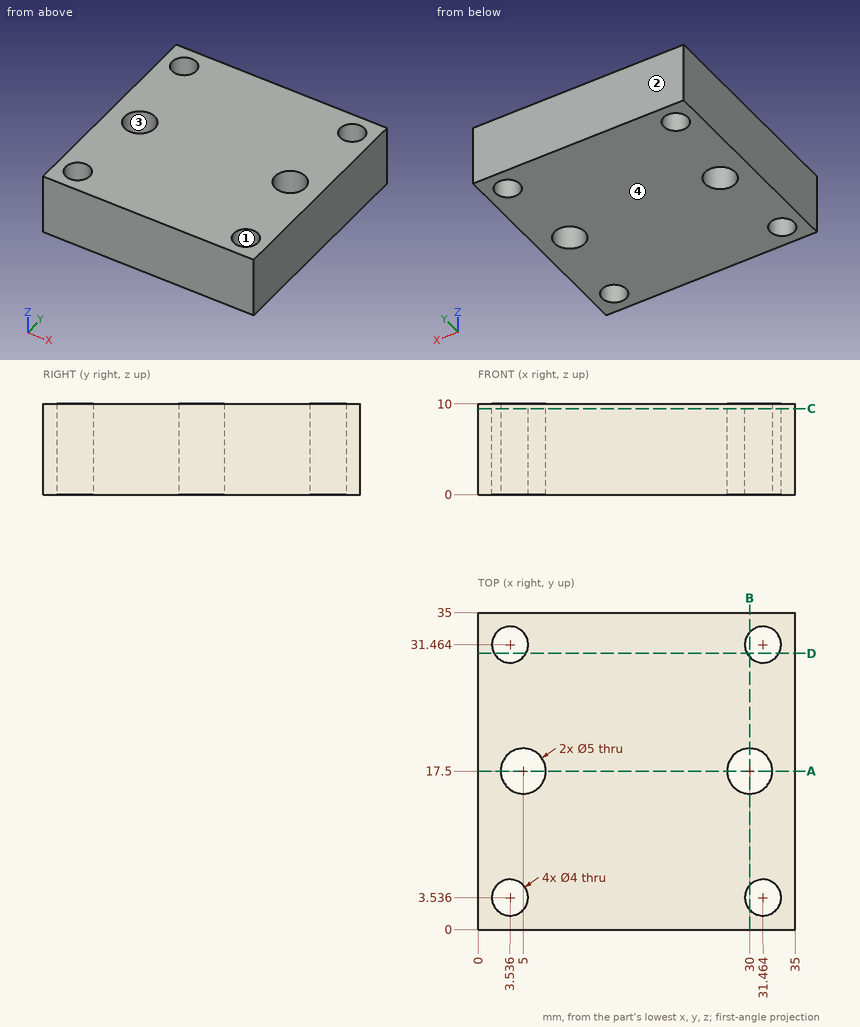
The figure shows three views and two pictorial views of one solid part (mm, origin at its lowest corner). Answer the questions. Give positions to 0.01 mm unless a question says otherwise; leave off trailing zeros. Order: outer loops, then holes, each group sorted by start corner. A loop starts at its lowest first (then second) coordinate and runs counter-clockwise, first axis right, second up. Notation, with made-up numbers: M 44.25,0.25 L 61.25,0.25 A25 cw 61.25,24.25 Z; hole C 46.25,11 d11. An arc over 180 degrees is marked long. Return JSON: item names as keys, results as strings.
Q1. This flat-tipped pin is pushed along its axis until it touches: pin 1 (3 mm diameter, centred on x = 30, y = 17.5, fed in from -Z). Where does it stop, or does it pass through?
Answer below:
{"pin 1": "passes through"}
Q2. Find section B-B, the plane x = 30. Write down the section's boundary in (y, z).
Answer below:
{"outline": "M 0,0 L 2.17,0 L 2.17,10 L 0,10 Z; M 4.9,0 L 15,0 L 15,10 L 4.9,10 Z; M 20,0 L 30.1,0 L 30.1,10 L 20,10 Z; M 32.83,0 L 35,0 L 35,10 L 32.83,10 Z"}
Q3. Find section A-A, the plane y = 17.5. Write down the section's boundary in (x, z).
Answer below:
{"outline": "M 0,0 L 2.5,0 L 2.5,10 L 0,10 Z; M 7.5,0 L 27.5,0 L 27.5,10 L 7.5,10 Z; M 32.5,0 L 35,0 L 35,10 L 32.5,10 Z"}
Q4. Find section D-D, the plane y = 30.5. Write down the section's boundary in (x, z), and give its area (3 significant figures).
Answer below:
{"outline": "M 0,0 L 1.78,0 L 1.78,10 L 0,10 Z; M 5.29,0 L 29.71,0 L 29.71,10 L 5.29,10 Z; M 33.22,0 L 35,0 L 35,10 L 33.22,10 Z", "area": "280 mm^2"}
Q5. Find the intervals of material crossed by line 1 along X through (y, z) = (31.5, 8) (1 decimal); line 2 along X through (y, z) = (16, 6); line 3 along Y through (x, z) = (30, 7) (1 decimal), in increasing order. Write a range as [from, to].
Answer below:
{"line 1": "x = [0, 1.5], [5.5, 29.5], [33.5, 35]", "line 2": "x = [0, 3], [7, 28], [32, 35]", "line 3": "y = [0, 2.2], [4.9, 15], [20, 30.1], [32.8, 35]"}
Q6. Find section C-C, the plane z = 9.5. Write down the section's boundary in (x, y) (1 decimal), and give its area (3 significant figures).
Answer below:
{"outline": "M 0,0 L 35,0 L 35,35 L 0,35 Z; hole C 3.5,3.5 d4; hole C 3.5,31.5 d4; hole C 5,17.5 d5; hole C 30,17.5 d5; hole C 31.5,3.5 d4; hole C 31.5,31.5 d4", "area": "1,140 mm^2"}
Q7. The mould has two halves that part along Y. Classify the marked faces 1, 2, 3 and 4: pulls with the +Y half, pulls with the -Y half, needs draft (parallel to the pull), parting line crosses it, or undercut.
Answer below:
{"face 1": "undercut", "face 2": "pulls with the +Y half", "face 3": "undercut", "face 4": "needs draft"}
